Verification items for this drawing (mm, ordinates from the low corner). A direction names the side the tool comes from. Coordinates: 2 decimals unless noted, no trailing zeros. Order: outer loops, then holes, each group sorted by start corner. A loop starts at its lowest first (then second) coordinate and runs counter-clockwise, first axis right, second up. Notation, with made-up numbers: M 72,59.25 L 115,59.25 A19 cw 115,69.25 Z; hole C 9,-14.75 d4. An arc over 180 degrees is marked long. Answer as a JSON object with one key per item and string values. Group by question number.
(1) Material ranges on line 1 (Y direction, x = 38, z = 21.5); line 2 (Z direction, x = 4, y = 9.5), recorded low to high.
(2) Access from +Z, -Z, +X, -X, +Y, -Y to the whole of each face (thin tool, end or side, straight path). Record for the marked faces 1, 2 and 3.
(3) Cross-section at B-B (x = 11). Enter the section's corners in (y, z).
(4) Gauge pin test, flat ends, axial feed: pin 1 Ø9.5 at (x, y) = (8.5, 11) entering from +Z; pin 2 Ø5.5 at (y, z) = (9.5, 22.5) entering from -X. Record the tip position at first contact, or that the pin passes through.
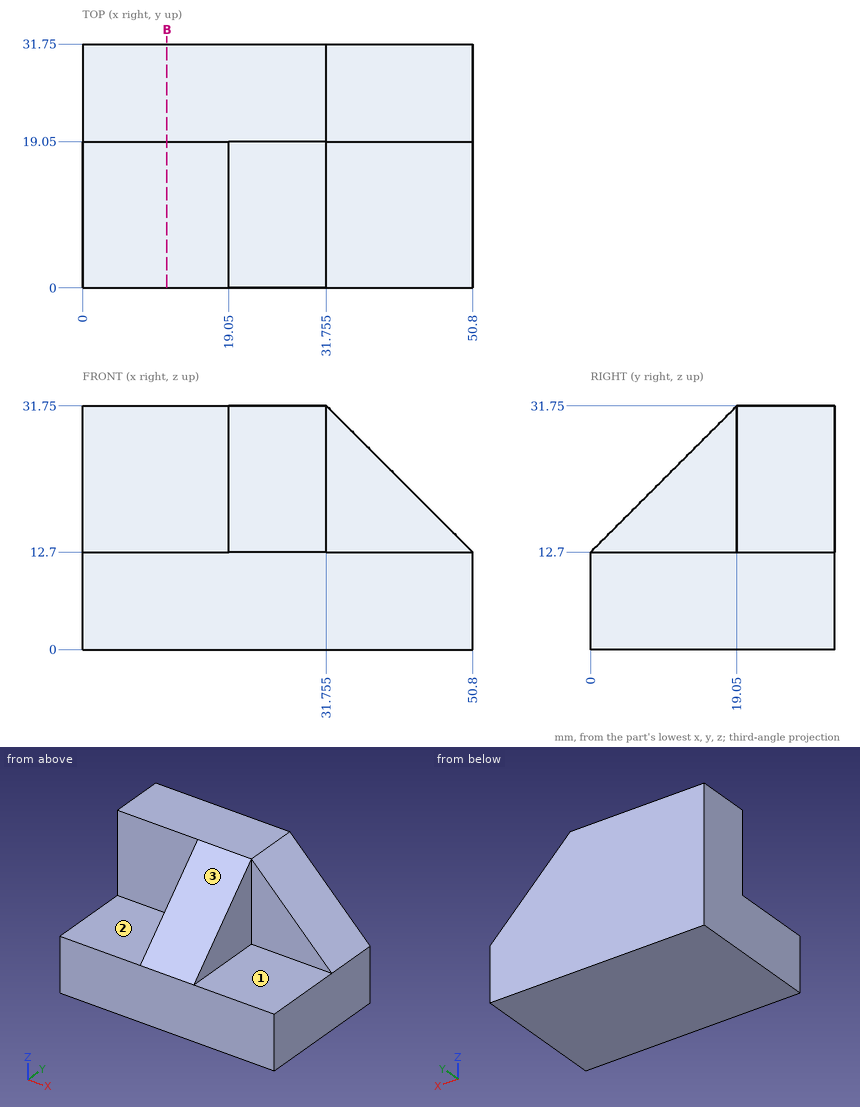
Taken from the geometry:
{
 "1": {"line 1": "y = 19.05 to 31.75", "line 2": "z = 0 to 12.7"},
 "2": {"face 1": "+Z, +X, -Y", "face 2": "+Z, -X, -Y", "face 3": "+Z, +X, -X, -Y"},
 "3": {"outline": "M 0,0 L 31.75,0 L 31.75,31.75 L 19.05,31.75 L 19.05,12.7 L 0,12.7 Z"},
 "4": {"pin 1": "stops at z = 12.7", "pin 2": "stops at x = 19.05"}
}
